```python
from build123d import *

# Parameters (mm, degrees)
BOSS_EXTRUDE1_DEPTH = 120
RIB6_REACH          = 89.955
SKETCH4_WALL_W      = 232.65925255
SKETCH4_WALL_H      = 6
CUT_EXTRUDE1_DEPTH  = 137.147387456
SCALE3_SCALE        = 7.5


with BuildPart() as part:
    # Sketch1 → Boss-Extrude1 (new body)
    with BuildSketch(Plane(origin=(0, 0, 0), x_dir=(1, 0, 0), z_dir=(0, 1, 0))):
        with BuildLine():
            Line((0, 0), (0, 32.333333333))
            ThreePointArc((0, 32.333333333), (0.292893219, 33.040440115), (1, 33.333333333))
            Line((1, 33.333333333), (5, 33.333333333))
            ThreePointArc((5, 33.333333333), (5.707106781, 33.040440115), (6, 32.333333333))
            Line((6, 32.333333333), (6, 7))
            ThreePointArc((6, 7), (6.292893219, 6.292893219), (7, 6))
            Line((7, 6), (54, 6))
            ThreePointArc((54, 6), (54.707106781, 5.707106781), (55, 5))
            Line((55, 5), (55, 1))
            ThreePointArc((55, 1), (54.707106781, 0.292893219), (54, 0))
            Line((54, 0), (0, 0))
        make_face()
    extrude(amount=BOSS_EXTRUDE1_DEPTH)

    # Sketch4 wall → Rib6 (add, up to next)
    with BuildSketch(Plane(origin=(30, 60, -19.166666666), x_dir=(0.876729593434, 0, 0.480983596392), z_dir=(0.480983596392, 0, -0.876729593434)), mode=Mode.PRIVATE) as rib6_sk1:
        Rectangle(SKETCH4_WALL_W, SKETCH4_WALL_H)
    rib6_tool1 = extrude(rib6_sk1.sketch, amount=-RIB6_REACH, mode=Mode.PRIVATE) - part.part
    add(rib6_tool1.solids().sort_by_distance((30, 60, -19.166666666))[0])

    # Sketch5 → Cut-Extrude1 (cut, through all)
    with BuildSketch(Plane.XY):
        Polygon((55, 120), (5, 120), (55, 90), align=None)
        Polygon((55, 30), (55, 0), (5, 0), align=None)
    extrude(amount=-CUT_EXTRUDE1_DEPTH, mode=Mode.SUBTRACT)


with BuildPart() as part_1:
    # Scale3: scaled about (16.387200979, 60, -9.868580773)
    add(part.part.scale(SCALE3_SCALE).moved(Location((-106.516806363, -390, 64.145775024))))


solid = part_1.part
```
Can you work these out from the model? Positions are in its coordinate system, mm. A direction names the side the tool comes from. Give positions to 0.01 mm unless a question says otherwise; leave off trailing zeros. Loops run counter-clockwise (first coordinate to the right, second up) from the corner with the lowest first, then second, coordinate; pieces in that order, holes last. Notation, with made-up numbers: M 46.5,-3 L 59.5,-3 A29 ccw 59.5,33 Z; hole C 2,-1 d3. An arc over 180 degrees is marked long. Use one line per item in the form item = value. Start each with the question number.
(1) On a 3-axis mill with a long thin cutter (end or side, diameter ignored), from which of +Z, -Z, +X, -X, +Y, -Y can I reach the whole of each face in a straight line? I mean faces 1 (the flat face through (-88, 510, -63)), 2 (the flat face through (-61.517, 291, -85)), 3 (the flat face through (-61.517, -177, -85)). Say none if no direction works.
(2) Please list where these lines run through material, in increasing order: line 1 (Y direction, x = -11.5, z = 13.5); line 2 (X direction, y = 209, z = 10.5); line 3 (Z direction, x = -0.5, y = 212).
(3) I want a section at A-A, the plane z = -16. Write out the boundary of the cut face in (x, y).
(4) I'm going to push flat-ended pins straight in: P1, Ø6, axis at x = 54, y = -39.5, coming from the -Z side; P2, Ø8, axis at x = -25.5, z = -131.5, coming from the +Y side; P3, Ø6, axis at x = -30.5, z = -22, coming from the -Y side. Where does each tip first touch, or does it pass through?
(5) I want a section at C-C, the plane x = 182. Write out the boundary of the cut face in (y, z), and give its area (3 significant figures).
(6) I want a section at B-B, the plane y = 152.5. Write out the boundary of the cut face in (x, z).
(7) I want a section at D-D, the plane z = -119.5. Write out the boundary of the cut face in (x, y), and give its area (3 significant figures).
Worked out:
q1.face_1 = +Z, -Z, +X, -X, +Y
q1.face_2 = -Z, +X, +Y
q1.face_3 = -Z, +X, -Y
q2.line_1 = 37.5 to 82.5
q2.line_2 = -106.52 to -61.52
q2.line_3 = 19.15 to 64.15
q3.outline = M -106.52,-390 L -69.02,-390 L -61.52,-385.5 L -61.52,37.5 L 234.42,37.5 L 234.42,82.5 L -61.52,82.5 L -61.52,505.5 L -69.02,510 L -106.52,510 Z
q4.P1 = 19.15
q4.P2 = 82.5
q4.P3 = 37.5
q5.outline = M -239.39,19.15 L 37.5,19.15 L 37.5,-44.76 L 82.5,-44.76 L 82.5,19.15 L 359.39,19.15 L 359.39,64.15 L -239.39,64.15 Z
q5.area = 29,800 mm²
q6.outline = M -106.52,-178.35 A7.5 ccw -99.02,-185.85 L -69.02,-185.85 A7.5 ccw -61.52,-178.35 L -61.52,11.65 A7.5 cw -54.02,19.15 L 298.48,19.15 A7.5 ccw 305.98,26.65 L 305.98,56.65 A7.5 ccw 298.48,64.15 L -106.52,64.15 Z
q7.outline = M -106.52,-390 L -69.02,-390 L -61.52,-385.5 L -61.52,37.5 L 45.76,37.5 L 45.76,82.5 L -61.52,82.5 L -61.52,505.5 L -69.02,510 L -106.52,510 Z
q7.area = 45,300 mm²
